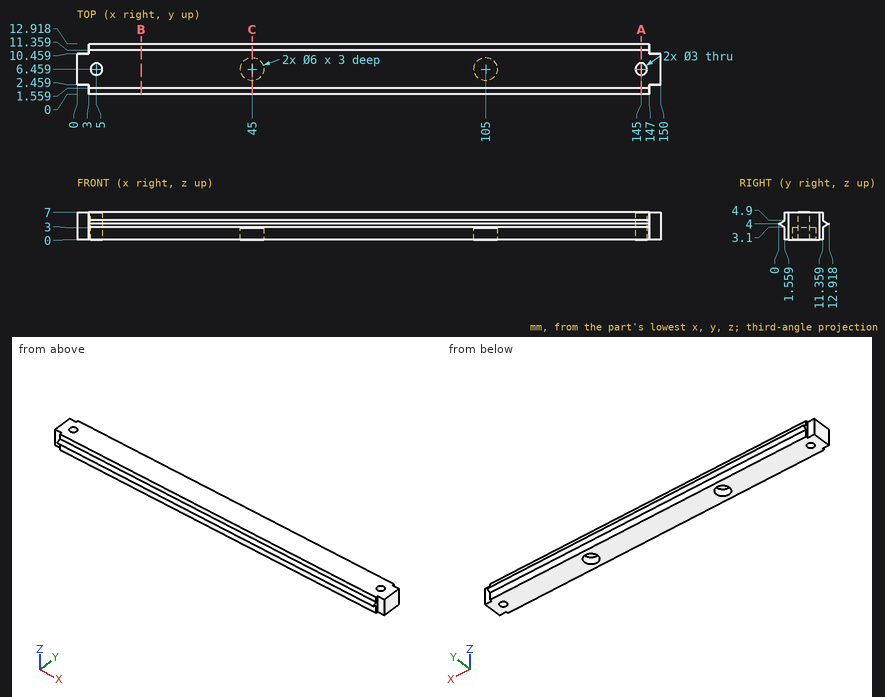
The figure shows three views and two pictorial views of one solid part (mm, origin at its lowest corner). Answer the questions. Round coordinates to 2 decimals unless told otherwise and drop trailing zeros. Order: outer loops, then holes, each group sorted by start corner. A loop starts at its lowest first (then second) coordinate and runs counter-clockwise, first axis right, second up. Notation, with made-up numbers: (-38.75, 50) -> (-21.75, 50) arc R18 cw to (-21.75, 59) -> close; hole circle Ø11 at (22, 46.5). An arc over 180 degrees is marked (long way). One line per item, written item: value.
Item 1: Find section B-B, the plane x = 16.5. Give the vertices of the cut face in (y, z).
Taken from the geometry:
outline: (0, 4) -> (1.56, 3.1) -> (1.56, 0) -> (11.36, 0) -> (11.36, 3.1) -> (12.92, 4) -> (11.36, 4.9) -> (11.36, 7) -> (1.56, 7) -> (1.56, 4.9) -> close
Item 2: Find section A-A, the plane x = 145. Give the vertices of the cut face in (y, z), then the cut area to 3 significant figures.
Taken from the geometry:
outline: (0, 4) -> (1.56, 3.1) -> (1.56, 0) -> (4.96, 0) -> (4.96, 7) -> (1.56, 7) -> (1.56, 4.9) -> close; (7.96, 0) -> (11.36, 0) -> (11.36, 3.1) -> (12.92, 4) -> (11.36, 4.9) -> (11.36, 7) -> (7.96, 7) -> close
area: 50.4 mm2
Item 3: Straight lines are drawn through the part: L1, parallel to X at y = 5.25, z = 2.5 (1 decimal); L2, parallel to Y at x = 108.5, z = 3; L3, parallel to Z at x = 103.5, y = 5.5. For each, find the intervals that lie inside material, in ascending order.
Taken from the geometry:
L1: x = 0 to 4.1, 5.9 to 42.3, 47.7 to 102.3, 107.7 to 144.1, 145.9 to 150
L2: y = 1.56 to 11.36
L3: z = 3 to 7
Item 4: Find section C-C, the plane x = 45. Give the vertices of the cut face in (y, z).
Taken from the geometry:
outline: (0, 4) -> (1.56, 3.1) -> (1.56, 0) -> (3.46, 0) -> (3.46, 3) -> (9.46, 3) -> (9.46, 0) -> (11.36, 0) -> (11.36, 3.1) -> (12.92, 4) -> (11.36, 4.9) -> (11.36, 7) -> (1.56, 7) -> (1.56, 4.9) -> close
Item 5: Given P1, Ø1.5, axis at x = 148, z = 2, coming from the +Y side; P2, Ø3, axis at x = 71, z = 4.5, coming from the +Y side; P3, Ø2.5, axis at x = 148.5, z = 2.5, coming from the -Y side, each flat-ended and moving along its own axis, determine where each tip first touches the part or whether it passes through.
Taken from the geometry:
P1: stops at y = 10.46
P2: stops at y = 12.92
P3: stops at y = 2.46
